from build123d import *

# Parameters (mm, degrees)
SKETCH1_R             = 5.42
BOSS_EXTRUDE1_DEPTH   = 2.03
BOSS_EXTRUDE1_2_DEPTH = 2.03
BOSS_EXTRUDE1_3_DEPTH = 2.03
BOSS_EXTRUDE1_4_DEPTH = 2.03
BOSS_EXTRUDE1_5_DEPTH = 2.03
BOSS_EXTRUDE2_DEPTH   = 2.03
SKETCH3_R             = 9
BOSS_EXTRUDE3_DEPTH   = 2.03


with BuildPart() as part:
    # Sketch1 → Boss-Extrude1 (new body)
    with BuildSketch(Plane.XY):
        with Locations((0, -32.53)):
            Circle(SKETCH1_R)
    extrude(amount=BOSS_EXTRUDE1_DEPTH)



with BuildPart() as body_2:
    # Sketch1 → Boss-Extrude1 2 (new body)
    with BuildSketch(Plane.XY):
        with Locations((-19.120654257, -26.317322827)):
            Circle(SKETCH1_R)
    extrude(amount=BOSS_EXTRUDE1_2_DEPTH)


with BuildPart() as body_3:
    # Sketch1 → Boss-Extrude1 3 (new body)
    with BuildSketch(Plane.XY):
        with Locations((-30.937868475, -10.052322827)):
            Circle(SKETCH1_R)
    extrude(amount=BOSS_EXTRUDE1_3_DEPTH)


with BuildPart() as body_4:
    # Sketch1 → Boss-Extrude1 4 (new body)
    with BuildSketch(Plane.XY):
        with Locations((-30.937868475, 10.052322827)):
            Circle(SKETCH1_R)
    extrude(amount=BOSS_EXTRUDE1_4_DEPTH)


with BuildPart() as body_5:
    # Sketch1 → Boss-Extrude1 5 (new body)
    with BuildSketch(Plane.XY):
        with Locations((-19.120654257, 26.317322827)):
            Circle(SKETCH1_R)
    extrude(amount=BOSS_EXTRUDE1_5_DEPTH)


with BuildPart() as part_1:
    add(part.part)

    add(body_2.part)  # Boss-Extrude2 merges body 2

    add(body_3.part)  # Boss-Extrude2 merges body 3

    add(body_4.part)  # Boss-Extrude2 merges body 4

    add(body_5.part)  # Boss-Extrude2 merges body 5
    # Sketch2 → Boss-Extrude2 (add)
    with BuildSketch(Plane.XY.offset(2.03)):
        with BuildLine():
            Line((-20.296224762, 27.935356816), (-17.945083752, 24.699288838))
            ThreePointArc((-17.945083752, 24.699288838), (-29.035755442, -9.434288838), (0, -30.53))
            Line((0, -30.53), (0, -34.53))
            ThreePointArc((0, -34.53), (-32.839981508, -10.670356816), (-20.296224762, 27.935356816))
        make_face()
    extrude(amount=-BOSS_EXTRUDE2_DEPTH)

    # Sketch3 → Boss-Extrude3 (add)
    with BuildSketch(Plane.XY.offset(2.03)):
        with Locations((-19.120654257, -26.317322827)):
            Circle(SKETCH3_R)
    extrude(amount=-BOSS_EXTRUDE3_DEPTH)


solid = part_1.part
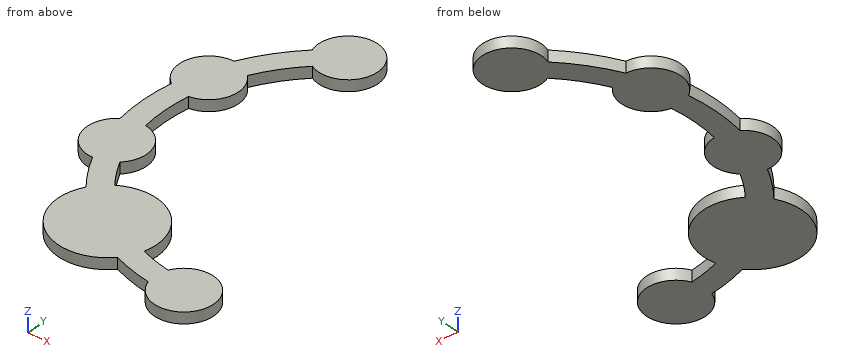
Verification items for the finished model (mm, model axes). Coordinates: 2 decimals unless noted, no trailing zeros. Loops run counter-clockwise (first coordinate to the right, second up) from the corner with the lowest first, then second, coordinate; pieces in that order, holes last. Notation, with made-up numbers: (9.25, 32.25) -> (21.25, 32.25) arc R5 cw to (21.25, 39.25) -> close; hole circle Ø6 at (73, 31.5). An arc over 180 degrees is marked (long way). Answer as CSV lines item,"result".
1) Cross-section at D-D, the plane y = 27. Record the cut outline in (x, z).
Found:
outline,"(-24.5, 0) -> (-13.74, 0) -> (-13.74, 2.03) -> (-24.5, 2.03) -> close"
2) Depth check by flat-ended pin: pin 1 (12 mm diameter, centred on x = -17.5, y = 10, fed in from -Z). Enter the tip coordinate at first touch or a pass-through.
Found:
pin 1,"passes through"
3) Thickness scan on L1, parallel to X at y = -18.5, z = 0.2; L2, parallel to Y at x = -23, z = 1.5; L3, parallel to X at y = 0.5, z = 1.15. Record the ranges inside material, lowest first. Write a range as from..to.
Found:
L1,"x = -29.16..-24.29, -23.58..-14.66"
L2,"y = -34.44..-18.2, 20.08..30.1"
L3,"x = -34.53..-30.53"
4) Cross-section at A-A, the plane x = -23. Record the cut outline in (y, z).
Found:
outline,"(-34.44, 0) -> (-18.2, 0) -> (-18.2, 2.03) -> (-34.44, 2.03) -> close; (20.08, 0) -> (30.1, 0) -> (30.1, 2.03) -> (20.08, 2.03) -> close"
5) Cross-section at B-B, the plane z = 1. Record the cut outline in (x, y).
Found:
outline,"(-34.07, -5.63) arc R5.42 ccw to (-30.87, -15.47) arc R34.53 ccw to (-26.85, -21.71) arc R9 ccw to (-12.35, -32.25) arc R34.53 ccw to (-5.18, -34.14) arc R5.42 ccw (long way) to (-4.86, -30.14) arc R30.53 cw to (-10.44, -28.69) arc R9 ccw to (-24.06, -18.79) arc R30.53 cw to (-27.16, -13.94) arc R5.42 ccw to (-30.17, -4.69) arc R30.53 cw to (-30.17, 4.69) arc R5.42 ccw to (-27.16, 13.94) arc R30.53 cw to (-21.65, 21.52) arc R5.42 ccw (long way) to (-24.25, 24.58) arc R34.53 ccw to (-30.87, 15.47) arc R5.42 ccw to (-34.07, 5.63) arc R34.53 ccw to start"
6) Cross-section at C-C, the plane x = 0. Record the cut outline in (y, z).
Found:
outline,"(-37.95, 0) -> (-27.11, 0) -> (-27.11, 2.03) -> (-37.95, 2.03) -> close"
